from build123d import *

# Parameters (mm, degrees)
SKETCH_1_W               = 39
SKETCH_1_H               = 39
EXTRUDE_1_DEPTH          = 22
SKETCH_2_R               = 11
EXTRUDE_2_DEPTH          = 2
SKETCH_3_R               = 2.5
EXTRUDE_3_DEPTH          = 17
CUT_EXTRUDE_1_DEPTH      = 5
CUT_EXTRUDE_1_DEPTH_BACK = 5
FILLET_1_R               = 0.5
CUT_EXTRUDE_2_DEPTH      = 36.277471565


# Read off the part's stored shape, not the designer's step: M3 螺纹孔1
with BuildPart() as part:
    # 草图1 → 凸台-拉伸1 (new body)
    with BuildSketch(Plane.XY):
        Rectangle(SKETCH_1_W, SKETCH_1_H)
    extrude(amount=EXTRUDE_1_DEPTH)

    # 草图2 → 凸台-拉伸2 (add)
    with BuildSketch(Plane.XY.offset(22)):
        Circle(SKETCH_2_R)
    extrude(amount=EXTRUDE_2_DEPTH)

    # 草图3 → 凸台-拉伸3 (add)
    with BuildSketch(Plane.XY.offset(24)):
        Circle(SKETCH_3_R)
    extrude(amount=EXTRUDE_3_DEPTH)

    # 草图5 → 切除-拉伸1 (cut, two sides: drawn at the far end of the back side and taken through both)
    with BuildSketch(Plane.XY.offset(11).offset(-CUT_EXTRUDE_1_DEPTH_BACK)):
        Polygon((13.496470179, 19.5), (19.5, 13.496470179), (19.5, 19.5), align=None)
        Polygon((19.5, -19.5), (13.49647018, -19.5), (19.5, -13.496470179), align=None)
        Polygon((-13.496470179, -19.5), (-19.5, -13.49647018), (-19.5, -19.5), align=None)
        Polygon((-19.5, 13.496470179), (-19.5, 19.5), (-13.496470179, 19.5), align=None)
    extrude(amount=CUT_EXTRUDE_1_DEPTH + CUT_EXTRUDE_1_DEPTH_BACK, mode=Mode.SUBTRACT)

    # 圆角1
    fillet_1_edges = [part.edges().sort_by_distance(p)[0] for p in [
        (-19.5, 0, 22),
        (-11, 0, 24),
        (0, -19.5, 22),
        (-2.5, 0, 41),
        (19.5, -19.5, 3),
        (-19.5, -19.5, 3),
        (-19.5, 19.5, 3),
        (19.5, 19.5, 3),
        (-19.5, 13.496470179, 11),
        (-13.496470179, 19.5, 11),
        (-16.49823509, 19.5, 6),
        (-19.5, 16.49823509, 6),
        (-16.49823509, 19.5, 16),
        (-19.5, 16.49823509, 16),
        (-16.49823509, -19.5, 6),
        (-13.496470179, -19.5, 11),
        (-19.5, -13.49647018, 11),
        (-19.5, -16.49823509, 6),
        (-16.49823509, -19.5, 16),
        (-19.5, -16.49823509, 16),
        (19.5, -16.49823509, 6),
        (19.5, -13.496470179, 11),
        (13.49647018, -19.5, 11),
        (16.49823509, -19.5, 6),
        (19.5, -16.49823509, 16),
        (16.49823509, -19.5, 16),
        (19.5, 0, 22),
        (0, -19.5, 0),
        (16.49823509, 19.5, 6),
        (13.496470179, 19.5, 11),
        (19.5, 13.496470179, 11),
        (19.5, 16.49823509, 6),
        (16.49823509, 19.5, 16),
        (19.5, 16.49823509, 16),
        (-19.5, 0, 0),
        (0, 19.5, 0),
        (19.5, 0, 0),
        (19.5, -19.5, 19),
        (-19.5, -19.5, 19),
        (-19.5, 19.5, 19),
        (19.5, 19.5, 19),
        (0, 19.5, 22),
    ]]
    fillet(fillet_1_edges, radius=FILLET_1_R)

    # 草图6 → 切除-拉伸2 (cut, through all)
    with BuildSketch(Plane.XY.offset(22)):
        Polygon((19.5, 19.5), (16.49823509, 19.5), (19.5, 16.49823509), align=None)
        Polygon((19.5, -19.5), (19.5, -16.49823509), (16.49823509, -19.5), align=None)
        Polygon((-19.5, -19.5), (-16.49823509, -19.5), (-19.5, -16.49823509), align=None)
        Polygon((-19.5, 19.5), (-19.5, 16.49823509), (-16.49823509, 19.5), align=None)
    extrude(amount=-CUT_EXTRUDE_2_DEPTH, mode=Mode.SUBTRACT)

    # M3 螺纹孔1 outline → M3 螺纹孔1 (revolve, cut)
    with BuildSketch(Plane(origin=(-15.5, 15.5, 0), x_dir=(1, 0, 0), z_dir=(0, -1, 0))):
        Polygon((0, 22), (0, 5.248924226), (1.25, 6), (1.25, 21.725), (1.525, 22), align=None)
    hole_wizard_m3_1 = revolve(axis=Axis((-15.5, 15.5, 0), (0, 0, 1)), mode=Mode.SUBTRACT)

    # Hole Wizard M3 _1 2 outline → Hole Wizard M3 _1 2 (revolve, cut)
    with BuildSketch(Plane(origin=(15.5, 15.5, 0), x_dir=(1, 0, 0), z_dir=(0, -1, 0))):
        Polygon((0, 22), (0, 5.248924226), (1.25, 6), (1.25, 21.725), (1.525, 22), align=None)
    hole_wizard_m3_1_2 = revolve(axis=Axis((15.5, 15.5, 0), (0, 0, 1)), mode=Mode.SUBTRACT)

    # 镜向1: M3 螺纹孔1, Hole Wizard M3 _1 2 across plane
    add(hole_wizard_m3_1.mirror(Plane.ZX), mode=Mode.SUBTRACT)
    add(hole_wizard_m3_1_2.mirror(Plane.ZX), mode=Mode.SUBTRACT)


solid = part.part
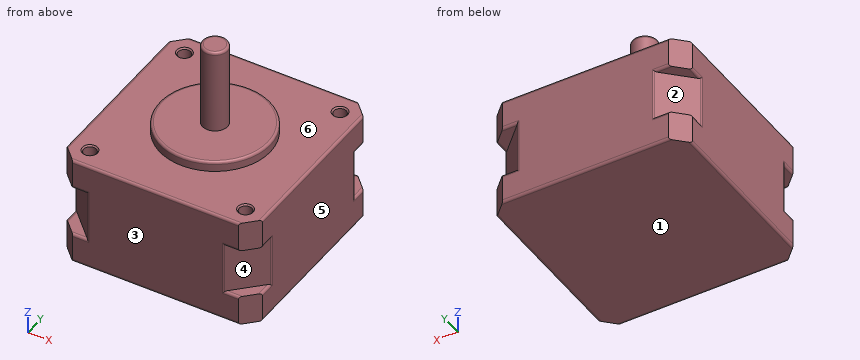
Geometry: final body of the model. Coordinates: model frame, mm. Face numbers are marked on the shaded views. A direction names the side the tool comes from. Give positions to 0.01 mm unless a question says otherwise; leave off trailing zeros. Write each loop counter-clockwise with the first axis right and the second up, starting at its lowest first coordinate (ties: lowest second). Pieces come first, ordered by that corner, then holes. Notation, with made-up numbers: (-5.75, -26) - (45.25, -26) arc R34 ccw to (45.25, 7) - close; hole circle Ø10 at (9, 24). An arc over 180 degrees is marked (long way). Return JSON: item names as keys, results as strings. Group by question number.
1) Set-up query: the marked faces 5 and 6. Return all of +Z, -Z, +X, -X, +Y, -Y with unobstructed straight access to the full face (end or side cutting, diameter ignored); none if empty.
2) Section B-B on y = 0. Return the cut outline in (x, z), plus the area to 3 significant figures.
3) Section A-A on z = 10.5. Return the cut outline in (x, y), plus the area to 3 significant figures.
4) Mould query, pull axis Z, two halves, no side actions, for the marked faces 1, 2, 3 and 4. Classes: released by +Z, released by -Z, zero draft, split by the parting line, or undercut.
5) First-contact query: P1, Ø10, axis at x = -13, y = 10, coming from the +Z side; P2, Ø2, axis at x = 15.5, y = -15.5, coming from the +Z side. Flat tips, straight axial feed; report the tip coordinate or a pass-through.
6) Line query: line 1 (Y direction, x = -15.5, z = 17.5); line 2 (X direction, y = -15.5, z = 15.5); line 3 (X direction, y = 15, z = 14). Output: solid intervals per line, ascending.
7) Section D-D on z = 29. Return the cut outline in (x, y).
Filled in:
{
 "1": {"face 5": "+Z, -Z, +X, +Y, -Y", "face 6": "+Z"},
 "2": {"outline": "(-19.5, 0.5) arc R0.5 ccw to (-19, 0) - (19, 0) arc R0.5 ccw to (19.5, 0.5) - (19.5, 21.5) arc R0.5 ccw to (19, 22) - (11, 22) - (11, 23.5) arc R0.5 ccw to (10.5, 24) - (2.5, 24) - (2.5, 40.5) arc R0.5 ccw to (2, 41) - (-2, 41) arc R0.5 ccw to (-2.5, 40.5) - (-2.5, 24) - (-10.5, 24) arc R0.5 ccw to (-11, 23.5) - (-11, 22) - (-19, 22) arc R0.5 ccw to (-19.5, 21.5) - close", "area": "987 mm^2"},
 "3": {"outline": "(-19.5, -13.29) arc R0.5 ccw to (-19.35, -13.64) - (-13.64, -19.35) arc R0.5 ccw to (-13.29, -19.5) - (13.29, -19.5) arc R0.5 ccw to (13.64, -19.35) - (19.35, -13.64) arc R0.5 ccw to (19.5, -13.29) - (19.5, 13.29) arc R0.5 ccw to (19.35, 13.64) - (13.64, 19.35) arc R0.5 ccw to (13.29, 19.5) - (-13.29, 19.5) arc R0.5 ccw to (-13.64, 19.35) - (-19.35, 13.64) arc R0.5 ccw to (-19.5, 13.29) - close; hole circle Ø2.5 at (-15.5, -15.5); hole circle Ø2.5 at (-15.5, 15.5); hole circle Ø2.5 at (15.5, -15.5); hole circle Ø2.5 at (15.5, 15.5)", "area": "1,430 mm^2"},
 "4": {"face 1": "released by -Z", "face 2": "undercut", "face 3": "zero draft", "face 4": "undercut"},
 "5": {"P1": "stops at z = 22", "P2": "stops at z = 5.85"},
 "6": {"line 1": "y = -19.5 to -16.75, -14.25 to 14.25, 16.75 to 19.5", "line 2": "x = -17.5 to -16.75, -14.25 to 14.25, 16.75 to 17.5", "line 3": "x = -18 to -16.65, -14.35 to 14.35, 16.65 to 18"},
 "7": {"outline": "circle Ø5 at (0, 0)"}
}
